Geometry check sheet. Reference: the model listing, model coordinates, mm. A direction names the side the tool comes from. Coordinates: 2 decimals unless noted, no trailing zeros. Order: outer loops, then holes, each group sorted by start corner. A loop starts at its lowest first (then second) coordinate and runs counter-clockwise, first axis right, second up. Notation, with made-up numbers: M 77.5,81 L 133.5,81 A7 ccw 133.5,87 Z; hole C 74,46 d10. An arc over 180 degrees is marked long. One line per item, written item: value. Start each with the question number.
1) Sectioned sample at C-C, the plane z = -48.5. Enter the section's corners in (x, y), then the cut area to 3 significant figures.
2) Sectioned sample at B-B, the plane x = -43.5. Enter the section's corners in (y, z).
3) Go/stop test with flat-tipped pins: P1, Ø4, axis at x = -33.5, y = -0.5, coming from the -Z side; P2, Ø10, axis at x = -27.5, y = 0, coming from the -Z side; P3, Ø3, axis at x = -16.5, y = -2.5, coming from the +Z side. Record where each tip stops, or that it passes through.
4) Access from +Z, -Z, +X, -X, +Y, -Y to the whole of each face (thin tool, end or side, straight path). Record for faces 5 (the flat face through (-42, -2.5, -51)), 6 (the flat face through (-23, 0, -41.131)), 7 (the flat face through (-2, -5.1, -51)).
5) Thickness scan on L1, parallel to X at y = -6.5, z = -36; L2, parallel to X at y = 1, z = -50; L3, parallel to X at y = 0, z = -67. Record the ranges inside material, lowest first. Write a range as from..to.
6) Sectioned sample at A-A, the plane z = -64. Enter the section's corners in (x, y), then the cut area to 3 significant figures.
7) Draft check along X on faces 1 (the flat face through (-2, 5.1, -51)), 2 (the flat face through (-34.98, 0, -66)), 3 (the flat face through (35, 0, -31.131)), 4 (the flat face through (-49.98, 0, -51)). Enter one of: pulls with the +X half, pulls with the -X half, needs draft (parallel to the pull), parting line crosses it, or undercut.
8) Sectioned sample at D-D, the plane y = 0. State how many separate pieces and enclosed holes the cut face has, then the cut area to 3 significant figures.
Autodesk Inventor part; units mm, degrees
ref_plane "YZ Plane" through (0, 0, 0) normal (1, 0, 0) x (0, 1, 0)
ref_plane "XZ Plane" through (0, 0, 0) normal (0, 1, 0) x (-1, 0, 0)
ref_plane "XY Plane" through (0, 0, 0) normal (0, 0, 1) x (1, 0, 0)
sketch "Sketch1" plane through (0, 0, 0) normal (0, 1, 0) x (-1, 0, 0)
  line L0 (41.98, 54.6032) -> (41.98, -104.2857) construction
  line L1 (-38.02, 54.6032) -> (-38.02, -101.9048) construction
  line L2 (49.98, -31.1313) -> (-46.02, -31.1313)
  line L3 (-46.02, -31.1313) -> (-46.02, -71.1313)
  line L4 (-46.02, -71.1313) -> (49.98, -71.1313)
  line L5 (49.98, -71.1313) -> (49.98, -31.1313)
  line L6 (1.98, 80.3555) -> (1.98, -108.9591)
  point P0 (0, 0)
  dimension "d0" = 80
  dimension "d1" = 8
  dimension "d2" = 40
extrude "Extrusion1" add sketch "Sketch1" along normal mid plane 20
sketch "Sketch2" plane through (46.02, 10, -71.1313) normal (0, 0, -1) x (-1, 0, 0)
  circle A0 centre (88, -10) radius 2.5 construction
  circle A1 centre (8, -10) radius 2.5 construction
  line L0 (10.5, -7.5) -> (5.5, -7.5)
  line L1 (5.5, -7.5) -> (5.5, -12.5)
  line L2 (5.5, -12.5) -> (10.5, -12.5)
  line L3 (10.5, -12.5) -> (10.5, -7.5)
  line L4 (85.5, -7.5) -> (90.5, -7.5)
  line L5 (90.5, -7.5) -> (90.5, -12.5)
  line L6 (90.5, -12.5) -> (85.5, -12.5)
  line L7 (85.5, -12.5) -> (85.5, -7.5)
  point P0 (46.02, -10)
  point P1 (88, -10)
  point P2 (8, -10)
  dimension "d5" = 5
  dimension "d6" = 5
extrude "Extrusion2" cut sketch "Sketch2" against normal through all
sketch "Sketch3" plane through (0, 10, 0) normal (0, 1, 0) x (1, 0, 0)
  line L0 (-49.98, 31.1313) -> (46.02, 31.1313) construction
  line L1 (46.02, 31.1313) -> (46.02, 71.1313) construction
  line L2 (46.02, 71.1313) -> (-49.98, 71.1313) construction
  line L3 (-49.98, 71.1313) -> (-49.98, 31.1313) construction
  line L4 (-34.98, 79.1313) -> (31.02, 79.1313)
  line L5 (31.02, 79.1313) -> (31.02, 61.1313)
  line L6 (31.02, 61.1313) -> (-34.98, 61.1313)
  line L7 (-34.98, 61.1313) -> (-34.98, 79.1313)
  line L8 (46.02, 31.1313) -> (-49.98, 31.1313) construction
  line L9 (-1.98, 31.1313) -> (-1.98, 128.9069) construction
  line L10 (-41.98, -54.6032) -> (-41.98, 104.2857) construction
  line L11 (-34.98, 23.1313) -> (31.02, 23.1313)
  line L12 (31.02, 23.1313) -> (31.02, 41.1313)
  line L13 (31.02, 41.1313) -> (-34.98, 41.1313)
  line L14 (-34.98, 41.1313) -> (-34.98, 23.1313)
  point P0 (0, 0)
  dimension "d9" = 7
  dimension "d10" = 10
  dimension "d11" = 18
  dimension "d14" = 10
  dimension "d15" = 18
extrude "Extrusion3" cut sketch "Sketch3" against normal through all
sketch "Sketch4" plane through (31.02, 10, -61.1313) normal (0, 0, -1) x (-1, 0, 0)
  line L0 (31.02, -10) -> (61.64, -10) construction
  line L1 (43, 0) -> (23, 0)
  line L2 (23, 0) -> (23, -20)
  line L3 (23, -20) -> (43, -20)
  line L4 (43, -20) -> (43, 0)
  line L5 (66, -20) -> (0, -20) construction
  line L6 (66, 0) -> (66, -20) construction
  line L7 (0, 0) -> (66, 0) construction
  line L8 (0, 0) -> (0, -20) construction
  line L9 (66, -20) -> (0, -20) construction
  line L10 (33, -20) -> (33, -66.7058) construction
  line L11 (66, -10) -> (82.2472, -10) construction
  dimension "d16" = 20
extrude "Extrusion4" add sketch "Sketch4" along normal blind 12 and the other way blind 40.5
ref_plane "Work Plane1" through (31.02, 10, -71.1313) normal (0, 0, -1) x (-1, 0, 0)
sketch "Sketch5" plane through (31.02, 10, -71.1313) normal (0, 0, -1) x (-1, 0, 0)
  line L0 (43, 0) -> (23, 0) construction
  line L1 (23, 0) -> (23, -20) construction
  line L2 (23, -20) -> (43, -20) construction
  line L3 (43, -20) -> (43, 0) construction
  line L4 (38.1, -4.9) -> (27.9, -4.9)
  line L5 (27.9, -4.9) -> (27.9, -15.1)
  line L6 (27.9, -15.1) -> (38.1, -15.1)
  line L7 (38.1, -15.1) -> (38.1, -4.9)
  line L8 (43, 0) -> (23, 0) construction
  line L9 (33, 0) -> (33, -20) construction
  line L10 (43, -20) -> (43, 0) construction
  line L11 (43, -10) -> (23, -10) construction
  line L12 (23, 0) -> (23, -20) construction
  point P0 (31.02, -10)
  dimension "d28" = 10.2
extrude "Extrusion5" cut sketch "Sketch5" against normal through all
ref_plane "Work Plane2" through (31.02, 10, -30.6313) normal (0, 0, -1) x (-1, 0, 0)
sketch "Sketch6" plane through (31.02, 10, -20.6313) normal (0, 0, 1) x (1, 0, 0)
  line L0 (-38.1, -25.1) -> (-27.9, -25.1)
  line L1 (-27.9, -25.1) -> (-27.9, 5.1)
  line L2 (-27.9, 5.1) -> (-38.1, 5.1)
  line L3 (-38.1, 5.1) -> (-38.1, -25.1)
  line L4 (-38.1, -4.9) -> (-27.9, -4.9) construction
  line L5 (-38.1, -15.1) -> (-38.1, -4.9) construction
  line L6 (-27.9, -15.1) -> (-38.1, -15.1) construction
  line L7 (-27.9, -4.9) -> (-27.9, -15.1) construction
  line L8 (-38.1, -15.1) -> (-38.1, -4.9) construction
  line L9 (-27.9, -4.9) -> (-27.9, -15.1) construction
  point P0 (-31.02, -10)
  dimension "d29" = 10
  dimension "d30" = 10
extrude "Extrusion6" cut sketch "Sketch6" against normal up to surface (10 mm away)
sketch "Sketch7" plane through (-11.98, -10, -41.1313) normal (-1, 0, 0) x (0, 0, 1)
  line L0 (10.5, -4) -> (10.5, 24) construction
  line L1 (0, 0) -> (0, 20) construction
  line L2 (20.5, 0) -> (0, 0) construction
  line L3 (20.5, 20) -> (20.5, 0) construction
  line L4 (0, 20) -> (20.5, 20) construction
  line L5 (20.5, 0) -> (20.5, 20) construction
  line L6 (20.5, 10) -> (1.9837, 10) construction
  line L7 (10.5, 0) -> (20.5, 0) construction
  line L8 (15.5, 0) -> (15.5, 20) construction
  line L9 (0, 20) -> (20.5, 20) construction
  circle A0 centre (15.5, 10) radius 1.5 construction
  line L10 (14, 8.5) -> (17, 8.5)
  line L11 (17, 8.5) -> (17, 11.5)
  line L12 (17, 11.5) -> (14, 11.5)
  line L13 (14, 11.5) -> (14, 8.5)
  point P0 (41.1313, 10)
  dimension "d31" = 3
extrude "Extrusion7" cut sketch "Sketch7" against normal through all
sketch "Sketch8" plane through (31.02, 10, -73.1313) normal (0, 0, -1) x (-1, 0, 0)
  line L0 (43, 0) -> (23, 0) construction
  line L1 (23, 0) -> (23, -20) construction
  line L2 (23, -20) -> (43, -20) construction
  line L3 (43, -20) -> (43, 0) construction
  line L4 (43, -10) -> (23, -10) construction
  line L5 (23, 0) -> (23, -20) construction
  line L6 (23, -20) -> (43, -20) construction
  line L7 (33, -20) -> (33, 0) construction
  circle A0 centre (33, -10) radius 2 construction
  line L8 (35, -12) -> (31, -12)
  line L9 (31, -12) -> (31, -8)
  line L10 (31, -8) -> (35, -8)
  line L11 (35, -8) -> (35, -12)
  point P0 (31.02, -10)
  dimension "d34" = 4
extrude "Extrusion8" cut sketch "Sketch8" against normal blind 20
equation "\"d6\" = d5"
properties part number "PRING_piston"
Final values:
1. outline: M -49.98,-10 L 46.02,-10 L 46.02,10 L -49.98,10 Z; hole M -44.48,-2.5 L -39.48,-2.5 L -39.48,2.5 L -44.48,2.5 Z; hole M -7.08,-5.1 L 3.12,-5.1 L 3.12,5.1 L -7.08,5.1 Z; hole M 35.52,-2.5 L 40.52,-2.5 L 40.52,2.5 L 35.52,2.5 Z
1. area: 1,770 mm^2
2. outline: M -10,-71.13 L -2.5,-71.13 L -2.5,-31.13 L -10,-31.13 Z; M 2.5,-71.13 L 10,-71.13 L 10,-31.13 L 2.5,-31.13 Z
3. P1: stops at z = -71.13
3. P2: stops at z = -61.13
3. P3: stops at z = -41.13
4. face 5: +Z, -Z
4. face 6: +Z, +Y, -Y
4. face 7: +Z
5. L1: x = -49.98..-34.98, -11.98..8.02, 31.02..46.02
5. L2: x = -49.98..-44.48, -39.48..-7.08, 3.12..35.52, 40.52..46.02
5. L3: x = -49.98..-44.48, -39.48..-34.98, -11.98..-7.08, 3.12..8.02, 31.02..35.52, 40.52..46.02
6. outline: M -49.98,-10 L -34.98,-10 L -34.98,10 L -49.98,10 Z; M -11.98,-10 L 8.02,-10 L 8.02,10 L -11.98,10 Z; M 31.02,-10 L 46.02,-10 L 46.02,10 L 31.02,10 Z; hole M -44.48,-2.5 L -39.48,-2.5 L -39.48,2.5 L -44.48,2.5 Z; hole M -7.08,-5.1 L 3.12,-5.1 L 3.12,5.1 L -7.08,5.1 Z; hole M 35.52,-2.5 L 40.52,-2.5 L 40.52,2.5 L 35.52,2.5 Z
6. area: 846 mm^2
7. face 1: undercut
7. face 2: undercut
7. face 3: needs draft
7. face 4: pulls with the -X half
8. separate pieces: 6
8. enclosed holes: 0
8. area: 2,220 mm^2
